```python
from build123d import *

# Parameters (mm, degrees)
SKETCH1_W            = 126.5
SKETCH1_H            = 192.5
BOSS_EXTRUDE1_DEPTH  = 3
CUT_EXTRUDE1_REACH   = 117.211
SKETCH2_R            = 8.25
M3_CLEARANCE_HOLE1_D = 3.4
FILLET1_R            = 3
M3_TAPPED_HOLE1_D    = 2.46


with BuildPart() as part:
    # Sketch1 → Boss-Extrude1 (new body)
    with BuildSketch(Plane(origin=(0, 0, 0), x_dir=(1, 0, 0), z_dir=(0, 1, 0))):
        Rectangle(SKETCH1_W, SKETCH1_H)
    extrude(amount=BOSS_EXTRUDE1_DEPTH)

    # Sketch2 → Cut-Extrude1 (cut, up to next)
    with BuildSketch(Plane(origin=(0, 3, 0), x_dir=(1, 0, 0), z_dir=(0, 1, 0)), mode=Mode.PRIVATE) as cut_extrude1_sk1:
        with Locations((67, 0)):
            Circle(SKETCH2_R)
    cut_extrude1_tool1 = extrude(cut_extrude1_sk1.sketch, amount=-CUT_EXTRUDE1_REACH, mode=Mode.PRIVATE) & part.part
    cut_extrude1 = cut_extrude1_tool1.solids().sort_by_distance((67, 3, 0))[0]
    add(cut_extrude1, mode=Mode.SUBTRACT)

    # Mirror1: Cut-Extrude1 across plane
    add(cut_extrude1.mirror(Plane(origin=(0, 0, 0), x_dir=(0, 0, 1), z_dir=(1, 0, 0))), mode=Mode.SUBTRACT)

    # M3 Clearance Hole1 (through all)
    with Locations(Plane(origin=(0, 3, 0), x_dir=(1, 0, 0), z_dir=(0, 1, 0))):
        with Locations((-57.75, 90.75), (57.75, -90.75), (57.75, 90.75), (-57.75, -90.75)):
            Hole(M3_CLEARANCE_HOLE1_D / 2)

    # Fillet1
    fillet1_edges = [part.edges().sort_by_distance(p)[0] for p in [
        (63.25, 1.5, 96.25),
        (-63.25, 1.5, 96.25),
        (-63.25, 1.5, -96.25),
        (63.25, 1.5, -96.25),
    ]]
    fillet(fillet1_edges, radius=FILLET1_R)

    # M3 Tapped Hole1 (through all)
    with Locations(Plane(origin=(0, 0, 0), x_dir=(-1, 0, 0), z_dir=(0, -1, 0))):
        with Locations((-6.773037989, -52.5), (-42.49999882, 83.49999962), (42.50000136, 19.50000062), (-6.773037989, -3.5), (51.226962011, -3.5), (51.226962011, -52.5)):
            Hole(M3_TAPPED_HOLE1_D / 2)


solid = part.part
```
Verification items for the finished model (mm, model axes). Give positions to 0.01 mm unless a question says otherwise; leave off trailing zeros. Loops run counter-clockwise (first coordinate to the right, second up) from the corner with the lowest first, then second, coordinate; pieces in that order, holes last. Notation, with made-up numbers: M 65.5,-19.75 L 105.5,-19.75 A30 ccw 105.5,16.25 Z; hole C 1.25,29 d8. An arc over 180 degrees is marked long. Return JSON: item names as keys, results as strings.
1) Mould release check, pull along Z, two halves, no side actions. Record for faces 1 (the flat face through (-1, 3, -1)), 2 (the cylindrical face through (58.75, 1.52, -0.13)): released by +Z, released by -Z, zero draft, split by the parting line, or undercut.
Findings:
{"face 1": "zero draft", "face 2": "undercut"}
2) Material ranges on L1, parallel to Z at x = -57.75, y = 0.9; L2, parallel to Z at x = 7, y = 1.4; L3, parallel to X at y = 1.6, z = 52.5, recorded low to high. Write a range as [from, to].
Findings:
{"L1": "z = [-96.25, -92.45], [-89.05, 89.05], [92.45, 96.25]", "L2": "z = [-96.25, 2.29], [4.71, 51.29], [53.71, 96.25]", "L3": "x = [-63.25, -52.46], [-50, 5.54], [8, 63.25]"}
3) Section check A-A, the plane z = -1. Enter the section's corners in (x, y).
Findings:
{"outline": "M -58.81,0 L 58.81,0 L 58.81,3 L -58.81,3 Z"}
